Part model, mm, in its own coordinate system. A direction names the side the tool comes from. Round coordinates to 2 decimals unless told otherwise and drop trailing zeros. Write each loop counter-clockwise with the first axis right and the second up, starting at its lowest first coordinate (ties: lowest second). Pieces come first, ordered by that corner, then holes. Notation, with made-up numbers: M 37.5,-15.75 L 90.5,-15.75 A24 ccw 90.5,15.25 Z; hole C 35.5,13.5 d8. An arc over 180 degrees is marked long. Use one line per item in the form item = value. Start each with the question number.
Item 1: Cut at D-D, the plane y = 15.5. Give the cut face in (x, z).
Item 2: Flat gauge pins, fed straight in: pin 1 Ø8 at (y, z) = (23.5, 6) entering from -X; pin 2 Ø6 at (x, y) = (29, 22) entering from +Z; pin 3 Ø12.5 at (x, y) = (79.5, 5) entering from +Z; pin 4 Ø23 at (x, y) = (-43.99, 6.35) entering from +Z. Where does each tip first touch, or does it go through?
Item 3: Mould opens along X. For faces 1 (the face through (80, 12.2, 31.75)), 2 (the face through (20.532, -12.693, 12.522)), 3 (the face through (-12.24, 6.21, 12.52)) say: +X half, -X half, draft (parallel to the pull), parting line (faces both ways), or undercut.
Item 4: Cut at B-B, the plane y = 9. Give the cut face in (x, z).
Item 5: Probe L1, parallel to X at y = 6, z = 9; L2, parallel to X at y = -2.5, z = 26; L3, parallel to Z at x = 89.5, y = 16.5. List the from-to ranges inside material, lowest first.
Item 6: Which spindle directions (+Z, -Z, +X, -X, +Y, -Y) get a long thin tool onto all of the face, cutting with end or side? Do faces 4 (the face through (19, 12.7, 13)), 5 (the face through (-69.37, 7.47, 23.02)), 6 (the face through (22.292, 25.216, 12.522)). Say none if no direction does.
Item 7: Cut at C-C, the plane z = 11. Give the cut face in (x, y), then the cut area to 3 significant figures.
Item 8: Cut at A-A, the plane x = 29.5. Give the cut face in (y, z).
from build123d import *

# Parameters (mm, degrees)
F0_R     = 19.05
F0_R_2   = 6.35
F1_DEPTH = 25.4
F2_R     = 25.4
F2_R_2   = 19.05
F3_DEPTH = 12.7
F4_R     = 12.7
F4_R_2   = 6.35
F5_DEPTH = 6.35


with BuildPart() as f1:
    # F0 (on Top) → F1 (new body)
    with BuildSketch(Plane.XY):
        with BuildLine():
            ThreePointArc((-41.452724, -18.922681), (-25.15558, -10.688838), (-18.592724, 6.35))
            ThreePointArc((-18.592724, 6.35), (-25.15558, 23.388838), (-41.452724, 31.622681))
            ThreePointArc((-41.452724, 31.622681), (-69.392724, 6.35), (-41.452724, -18.922681))
        make_face()
        with Locations((-43.992724, 6.35)):
            Circle(F0_R, mode=Mode.SUBTRACT)
        with BuildLine():
            ThreePointArc((-41.452724, 31.622681), (-25.15558, 23.388838), (-18.592724, 6.35))
            ThreePointArc((-18.592724, 6.35), (-25.15558, -10.688838), (-41.452724, -18.922681))
            Line((-41.452724, -18.922681), (84.277276, -6.28634))
            ThreePointArc((84.277276, -6.28634), (70.307276, 6.35), (84.277276, 18.98634))
            Line((84.277276, 18.98634), (-41.452724, 31.622681))
        make_face()
        with BuildLine():
            ThreePointArc((-5.892724, 0), (-12.242724, 6.35), (-5.892724, 12.7))
            Line((-5.892724, 12.7), (44.907276, 12.7))
            ThreePointArc((44.907276, 12.7), (49.397404, 10.840128), (51.257276, 6.35))
            ThreePointArc((51.257276, 6.35), (49.397404, 1.859872), (44.907276, 0))
            Line((44.907276, 0), (-5.892724, 0))
        make_face(mode=Mode.SUBTRACT)
        with BuildLine():
            ThreePointArc((95.707276, 6.35), (92.425848, 14.869419), (84.277276, 18.98634))
            ThreePointArc((84.277276, 18.98634), (70.307276, 6.35), (84.277276, -6.28634))
            ThreePointArc((84.277276, -6.28634), (92.425848, -2.169419), (95.707276, 6.35))
        make_face()
        with Locations((83.007276, 6.35)):
            Circle(F0_R_2, mode=Mode.SUBTRACT)
    extrude(amount=F1_DEPTH)

    # F2 (on face) → F3 (join)
    with BuildSketch(Plane.XY.offset(25.4)):
        with Locations((-43.992724, 6.35)):
            Circle(F2_R)
        with Locations((-43.992724, 6.35)):
            Circle(F2_R_2, mode=Mode.SUBTRACT)
    extrude(amount=F3_DEPTH)

    # F4 (on face) → F5 (join)
    with BuildSketch(Plane.XY.offset(25.4)):
        with Locations((83.007276, 6.35)):
            Circle(F4_R)
        with Locations((83.007276, 6.35)):
            Circle(F4_R_2, mode=Mode.SUBTRACT)
    extrude(amount=F5_DEPTH)


solid = f1.part
Model answer:
q1.outline = M -67.69,0 L -60.7,0 L -60.7,38.1 L -67.69,38.1 Z; M -27.28,0 L 91.81,0 L 91.81,31.75 L 74.2,31.75 L 74.2,25.4 L -20.3,25.4 L -20.3,38.1 L -27.28,38.1 Z
q2.pin_1 = -65.72
q2.pin_2 = 25.4
q2.pin_3 = 31.75
q2.pin_4 = through
q3.face_1 = draft
q3.face_2 = +X half
q3.face_3 = undercut
q4.outline = M -69.25,0 L -62.86,0 L -62.86,38.1 L -69.25,38.1 Z; M -25.13,0 L -11.66,0 L -11.66,25.4 L -18.73,25.4 L -18.73,38.1 L -25.13,38.1 Z; M 50.68,0 L 77.24,0 L 77.24,31.75 L 70.59,31.75 L 70.59,25.4 L 50.68,25.4 Z; M 88.78,0 L 95.43,0 L 95.43,31.75 L 88.78,31.75 Z
q5.L1 = -69.39 to -63.04, -24.95 to -12.23, 51.25 to 76.67, 89.35 to 95.7
q5.L2 = -67.8 to -60.86, -27.12 to -20.18, 73.9 to 92.12
q5.L3 = 0 to 31.75
q6.face_4 = +Z, -Z
q6.face_5 = +Z
q6.face_6 = +Z, -Z, +X, +Y
q7.outline = M -41.45,-18.92 L 84.28,-6.29 A12.7 ccw 84.28,18.99 L -41.45,31.62 A25.4 ccw long Z; hole C -43.99,6.35 d38.1; hole M -5.89,0 L 44.91,0 A6.35 ccw 44.91,12.7 L -5.89,12.7 A6.35 ccw Z; hole C 83.01,6.35 d12.7
q7.area = 4,090 mm²
q8.outline = M -11.79,0 L 0,0 L 0,25.4 L -11.79,25.4 Z; M 12.7,0 L 24.49,0 L 24.49,25.4 L 12.7,25.4 Z
